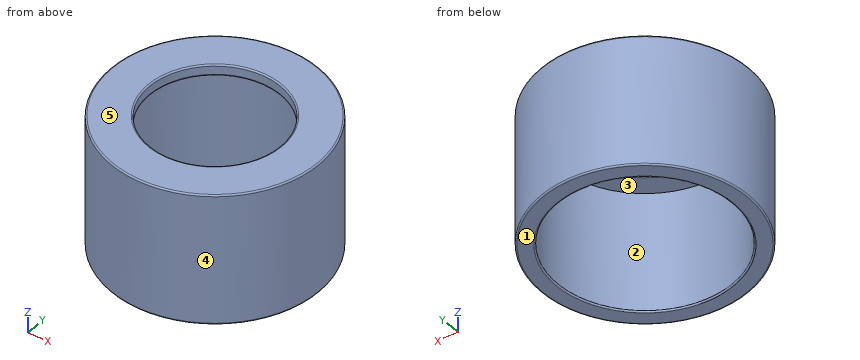
Autodesk Inventor part; units mm, degrees
ref_plane "YZ Plane" through (0, 0, 0) normal (1, 0, 0) x (0, 1, 0)
ref_plane "XZ Plane" through (0, 0, 0) normal (0, 1, 0) x (-1, 0, 0)
ref_plane "XY Plane" through (0, 0, 0) normal (0, 0, 1) x (1, 0, 0)
sketch "Sketch2" plane through (0, 0, 0) normal (0, 1, 0) x (-1, 0, 0)
  line L0 (6.4, -4.8) -> (7.6, -4.8)
  line L1 (7.6, -4.8) -> (7.6, 4.8)
  line L2 (7.6, 4.8) -> (4.8, 4.8)
  line L3 (4.8, 4.8) -> (4.8, 4)
  line L4 (4.8, 4) -> (6.4, 4)
  line L5 (6.4, 4) -> (6.4, -4.8)
  line L6 (0, 4.8) -> (0, -4.8)
  point P0 (0, 0)
  point P1 (0, 0)
  dimension "d0" = 15.2
  dimension "d1" = 9.6
  dimension "d2" = 0.8
  dimension "d3" = 9.6
  dimension "d4" = 12.8
revolve "Revolution1" add sketch "Sketch2" angle 360 about axis through (0, 0, 4.8) along (0, 0, -1)
fillet "Fillet1" radius 0.1 5 edges at (4.8, 0, 4.8) (4.8, 0, 4) (7.6, 0, 4.8) (7.6, 0, -4.8) (6.4, 0, -4.8)
equation "\"d1\" = lh"
equation "\"d3\" = lh"
properties part number "99401-RedRubber" material "Rubber"
Geometry: final body of the model. Coordinates: model frame, mm. Face numbers are marked on the shaded views. A direction names the side the tool comes from. Coordinates: 2 decimals unless noted, no trailing zeros. Loops run counter-clockwise (first coordinate to the right, second up) from the corner with the lowest first, then second, coordinate; pieces in that order, holes last. Notation, with made-up numbers: (-28.75, 56) -> (25.25, 56) arc R33 ccw to (25.25, 88) -> close; hole circle Ø1 at (-0.75, 85). An arc over 180 degrees is marked (long way). Use a Markdown table: item, result. Add a question column.
(1) Mould query, pull axis Y, two halves, no side actions, for the marked faces 3, 4 and 5. Classes: pulls with the +Y half, pulls with the -Y half, needs draft (parallel to the pull), parting line crosses it, or undercut.
(2) Access query for the marked faces 1 and 2. Directions: +Z, -Z, +X, -X, +Y, -Y. A direction counts if a zero-diameter tool reaches every point of the face in a straight line with its end or side. Return the directions, or none.
(3) Section query A-A, the plane x = 0. Return loops of the section in (y, z).
(4) Line query: line 1 along Y through (x, z) = (0, 4.5); line 2 along Y through (x, z) = (-0.5, -0.25); line 3 along X through (y, z) = (-4.75, 3.5). Output: solid intervals per line, ascending.
(5) Section query C-C, the plane z = 1.75. Return loops of the section in (x, y), plus the area to 3 significant figures.
(6) Pin query (flat end, axial travel): pin 1 Ø5 at (x, z) = (-4.5, 3.5) entering from -Y; pin 2 Ø5 at (x, z) = (6, -1.5) entering from +Y; pin 3 Ø2 at (x, z) = (5, 1) entering from +Y. Return the tip coordinate at first contact, or that it passes through.
Answer:
| question | item | result |
|---|---|---|
| 1 | face 3 | undercut |
| 1 | face 4 | parting line crosses it |
| 1 | face 5 | needs draft |
| 2 | face 1 | -Z, +X, -X, +Y, -Y |
| 2 | face 2 | -Z |
| 3 | outline | (-7.6, -4.7) arc R0.1 ccw to (-7.5, -4.8) -> (-6.5, -4.8) arc R0.1 ccw to (-6.4, -4.7) -> (-6.4, 4) -> (-4.9, 4) arc R0.1 ccw to (-4.8, 4.1) -> (-4.8, 4.7) arc R0.1 ccw to (-4.9, 4.8) -> (-7.5, 4.8) arc R0.1 ccw to (-7.6, 4.7) -> close; (4.8, 4.1) arc R0.1 ccw to (4.9, 4) -> (6.4, 4) -> (6.4, -4.7) arc R0.1 ccw to (6.5, -4.8) -> (7.5, -4.8) arc R0.1 ccw to (7.6, -4.7) -> (7.6, 4.7) arc R0.1 ccw to (7.5, 4.8) -> (4.9, 4.8) arc R0.1 ccw to (4.8, 4.7) -> close |
| 4 | line 1 | y = -7.6 to -4.8, 4.8 to 7.6 |
| 4 | line 2 | y = -7.58 to -6.38, 6.38 to 7.58 |
| 4 | line 3 | x = -5.93 to -4.29, 4.29 to 5.93 |
| 5 | outline | circle Ø15.2 at (0, 0); hole circle Ø12.8 at (0, 0) |
| 5 | area | 52.8 mm^2 |
| 6 | pin 1 | stops at y = -7.33 |
| 6 | pin 2 | stops at y = 6.75 |
| 6 | pin 3 | stops at y = 6.46 |
